from build123d import *

# Parameters (mm, degrees)
SKETCH1_W      = 30
SKETCH1_H      = 15
SKETCH1_H_2    = 5
EXTRUDE1_DEPTH = 8
EXTRUDE2_START = 5
SKETCH2_R      = 2
SKETCH2_W      = 30.8
SKETCH2_H      = 12
SKETCH2_W_2    = 22.8
SKETCH2_H_2    = 8
EXTRUDE2_DEPTH = 20
EXTRUDE3_START = 8
SKETCH3_W      = 28
SKETCH3_H      = 14
EXTRUDE3_DEPTH = 14
EXTRUDE4_DEPTH = 4
EXTRUDE5_START = -15
SKETCH2_3_W    = 22.8
SKETCH2_3_H    = 8
EXTRUDE5_DEPTH = 3
EXTRUDE6_START = -18
EXTRUDE6_DEPTH = 23


with BuildPart() as part:
    # Sketch1 → Extrude1 (new, symmetric)
    with BuildSketch(Plane.XY):
        Polygon((-15, 0), (-15, 5), (-23, 5), (-23, -1), (-18, -1), (-18, -18), (18, -18), (18, -1), (23, -1), (23, 5), (15, 5), (15, 0), (15, -15), (-15, -15), align=None)
        with Locations((0, -7.5)):
            Rectangle(SKETCH1_W, SKETCH1_H)
        with Locations((0, 2.5)):
            Rectangle(SKETCH1_W, SKETCH1_H_2)
    extrude(amount=EXTRUDE1_DEPTH, both=True)

    # Sketch2 → Extrude2 (cut)
    with BuildSketch(Plane(origin=(0, 0, 0), x_dir=(1, 0, 0), z_dir=(0, 1, 0)).offset(EXTRUDE2_START)):
        Polygon((-23, -8), (-23, -3.1), (-18.1, -8), align=None)
        with Locations(Location((-18.1, 0, 0), (0, 0, 272.865983983))):
            Circle(SKETCH2_R)
        Polygon((-23, 8), (-18.1, 8), (-23, 3.1), align=None)
        Rectangle(SKETCH2_W, SKETCH2_H)
        Rectangle(SKETCH2_W_2, SKETCH2_H_2, mode=Mode.SUBTRACT)
        Rectangle(SKETCH2_W_2, SKETCH2_H_2)
        Polygon((23, 3.1), (23, 8), (18.1, 8), align=None)
        with Locations(Location((18.1, 0, 0), (0, 0, 267.134016017))):
            Circle(SKETCH2_R)
        Polygon((18.1, -8), (23, -8), (23, -3.1), align=None)
    extrude(amount=-EXTRUDE2_DEPTH, mode=Mode.SUBTRACT)

    # Sketch3 → Extrude3 (cut)
    with BuildSketch(Plane.XY.offset(EXTRUDE3_START)):
        with Locations((0, -7)):
            Rectangle(SKETCH3_W, SKETCH3_H)
    extrude(amount=-EXTRUDE3_DEPTH, mode=Mode.SUBTRACT)

    # Sketch3<3> → Extrude4 (cut, symmetric)
    with BuildSketch(Plane.XY):
        Polygon((-14, -18), (-14, -14), (-14, -1), (-18, -1), (-18, -18), align=None)
        Polygon((14, -1), (14, -14), (14, -18), (18, -18), (18, -1), align=None)
    extrude(amount=EXTRUDE4_DEPTH, both=True, mode=Mode.SUBTRACT)

    # Sketch2<3> → Extrude5 (cut)
    with BuildSketch(Plane(origin=(0, 0, 0), x_dir=(1, 0, 0), z_dir=(0, 1, 0)).offset(EXTRUDE5_START)):
        Rectangle(SKETCH2_3_W, SKETCH2_3_H)
    extrude(amount=-EXTRUDE5_DEPTH, mode=Mode.SUBTRACT)

    # Sketch4 → Extrude6 (add)
    with BuildSketch(Plane(origin=(0, 0, 0), x_dir=(1, 0, 0), z_dir=(0, 1, 0)).offset(EXTRUDE6_START)):
        with BuildLine():
            Line((-18.1, 8), (-13.1, 8))
            Line((-13.1, 8), (-13.1, 13))
            ThreePointArc((-13.1, 13), (-14.564466094, 9.464466094), (-18.1, 8))
        make_face()
        Polygon((-13.1, 13), (-13.1, 8), (-10.486751346, 8), (-7.6, 13), align=None)
        Polygon((1.286751346, 8), (3.9, 8), (3.9, 13), (-1.6, 13), align=None)
        with BuildLine():
            Line((3.9, 13), (3.9, 8))
            Line((3.9, 8), (8.9, 8))
            ThreePointArc((8.9, 8), (5.364466094, 9.464466094), (3.9, 13))
        make_face()
    extrude(amount=EXTRUDE6_DEPTH)


solid = part.part
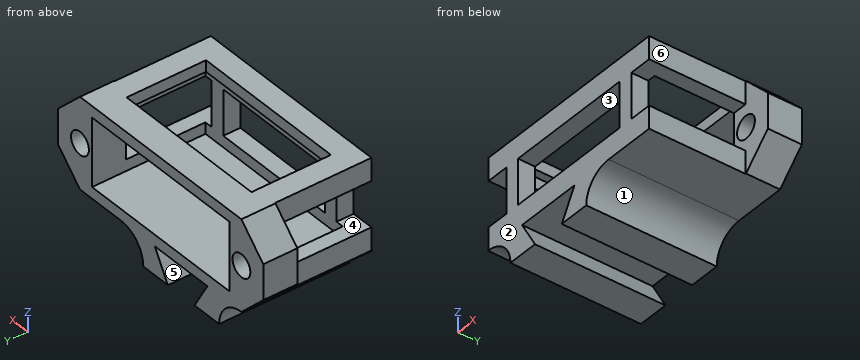
Input: part model. Units: mm. Frame: model coordinates. Face numbers are marked on the shaded views. A direction names the side the tool comes from. Give positions to 0.01 mm unless a question says otherwise; leave off trailing zeros. Loops run counter-clockwise (first coordinate to the right, second up) from the corner with the lowest first, then second, coordinate; pieces in that order, holes last. Notation, with made-up numbers: (-18.75, 72.5) -> (21.25, 72.5) arc R30 cw to (21.25, 95.5) -> close; hole circle Ø9 at (85, 53.25). An arc over 180 degrees is marked (long way). Answer as a JSON object with one key per item and string values. Group by question number.
Item 1: Reachability of the marked faces 4, 5 and 6 from +Z, -Z, +X, -X, +Y, -Y: full face, straight path, thin tool, end or side. Return the list, or none.
Item 2: Pull-direction query (X, two-part tool) for the marked faces 1, 2 and 3; classes: released by +X, released by -X, zero draft, split by the parting line, or undercut.
Item 3: Cut plane B-B, the plane z = 0. Return the cut outline in (x, y).
Item 4: Line query: probe 1 along X at (y, z) = (3.4, 0); probe 2 along Z at (x, y) = (18.1, 3.3); probe 3 along X at (y, z) = (-17, -1). Output: solid intervals per line, ascending.
Item 5: Cut plane C-C, the plane y = -2. Return the cut outline in (x, z).
Item 6: Pin query (flat end, axial travel): P1, Ø2, axis at x = 4.5, y = -5.5, coming from the +Z side; P2, Ø1.5, axis at x = 9.5, y = -3, coming from the -Z side; P3, Ø3, axis at y = -9.5, z = 6, coming from the +X side. Return the tip coordinate at first contact, or that it passes through.
Item 7: Cut plane D-D, the plane z = -7.25. Return the cut outline in (x, y).
Item 8: Cut plane A-A, the plane x = 2.5. Return the cut outline in (y, z), and give its area (3 significant figures).
Checks:
{
 "1": {"face 4": "-X, -Y", "face 5": "+Y, -Y", "face 6": "+Z, -Z, +X, -Y"},
 "2": {"face 1": "released by +X", "face 2": "zero draft", "face 3": "undercut"},
 "3": {"outline": "(-23, -1) -> (-20.1, -1) -> (-20.1, 5) -> (-23, 5) -> close; (-16.1, -1) -> (-15.4, -1) -> (-15.4, 5) -> (-16.1, 5) -> close; (-14, -18) -> (-11.4, -18) -> (-11.4, -15) -> (-14, -15) -> close; (11.4, -18) -> (14, -18) -> (14, -15) -> (11.4, -15) -> close; (15.4, -1) -> (16.1, -1) -> (16.1, 5) -> (15.4, 5) -> close; (20.1, -1) -> (23, -1) -> (23, 5) -> (20.1, 5) -> close"},
 "4": {"probe 1": "x = -23 to -20.1, -16.1 to -15.4, 15.4 to 16.1, 20.1 to 23", "probe 2": "z = -8 to -2, 2 to 8", "probe 3": "x = -14 to -11.4, 11.4 to 14"},
 "5": {"outline": "(-18.1, -8) arc R5 cw to (-13.1, -13) -> (-7.6, -13) -> (-10.49, -8) -> (1.29, -8) -> (-1.6, -13) -> (3.9, -13) arc R5 cw to (8.9, -8) -> (18, -8) -> (18, -4) -> (15.4, -4) -> (15.4, -6) -> (-15.4, -6) -> (-15.4, -4) -> (-18, -4) -> (-18, -8) -> close; (-18, 4) -> (-15.4, 4) -> (-15.4, 6) -> (-14, 6) -> (-14, 8) -> (-18, 8) -> close; (14, 6) -> (15.4, 6) -> (15.4, 4) -> (18, 4) -> (18, 8) -> (14, 8) -> close"},
 "6": {"P1": "stops at z = -6", "P2": "stops at z = -8", "P3": "stops at x = 18"},
 "7": {"outline": "(-18.85, -1) -> (-18, -1) -> (-18, -18) -> (18, -18) -> (18, -1) -> (18.85, -1) -> (18.85, 5) -> (-18.85, 5) -> close"},
 "8": {"outline": "(-18, -13) -> (5, -13) -> (5, -6) -> (-15, -6) -> (-15, -4) -> (-18, -4) -> close; (-18, 4) -> (-15, 4) -> (-15, 6) -> (-14, 6) -> (-14, 8) -> (-18, 8) -> close; (0, 6) -> (5, 6) -> (5, 8) -> (0, 8) -> close", "area": "191 mm²"}
}
